```python
from build123d import *

# Parameters (mm, degrees)
SKETCH1_R           = 3.175
SKETCH1_R_2         = 1.325
BOSS_EXTRUDE1_DEPTH = 8


with BuildPart() as part:
    # Sketch1 → Boss-Extrude1 (new body)
    with BuildSketch(Plane.XY):
        with BuildLine():
            Line((-21.75, 27.5), (-6, 27.5))
            ThreePointArc((-6, 27.5), (0, 36.5), (6, 27.5))
            Line((6, 27.5), (21.75, 27.5))
            Line((21.75, 27.5), (21.75, 19.489664619))
            Line((21.75, 19.489664619), (37.852514493, 8.977148354))
            Line((37.852514493, 8.977148354), (59.375273358, 15.378390657))
            Line((59.375273358, 15.378390657), (64.476863532, 23.056267795))
            ThreePointArc((64.476863532, 23.056267795), (74.130822267, 30.891394037), (70.5, 19))
            Line((70.5, 19), (64.476863532, 8.759983115))
            Line((64.476863532, 8.759983115), (64.476863532, -8.759983115))
            Line((64.476863532, -8.759983115), (70.5, -19))
            ThreePointArc((70.5, -19), (74.130822267, -30.891394037), (64.476863532, -23.056267795))
            Line((64.476863532, -23.056267795), (59.375273358, -15.378390657))
            Line((59.375273358, -15.378390657), (37.852514493, -8.977148354))
            Line((37.852514493, -8.977148354), (21.75, -19.489664619))
            Line((21.75, -19.489664619), (21.75, -27.5))
            Line((21.75, -27.5), (6, -27.5))
            ThreePointArc((6, -27.5), (0, -36.5), (-6, -27.5))
            Line((-6, -27.5), (-21.75, -27.5))
            Line((-21.75, -27.5), (-21.75, -19.489664619))
            Line((-21.75, -19.489664619), (-37.852514493, -8.977148354))
            Line((-37.852514493, -8.977148354), (-59.375273358, -15.378390657))
            Line((-59.375273358, -15.378390657), (-64.476863532, -23.056267795))
            ThreePointArc((-64.476863532, -23.056267795), (-74.130822267, -30.891394037), (-70.5, -19))
            Line((-70.5, -19), (-64.476863532, -8.759983115))
            Line((-64.476863532, -8.759983115), (-64.476863532, 8.759983115))
            Line((-64.476863532, 8.759983115), (-70.5, 19))
            ThreePointArc((-70.5, 19), (-74.130822267, 30.891394037), (-64.476863532, 23.056267795))
            Line((-64.476863532, 23.056267795), (-59.375273358, 15.378390657))
            Line((-59.375273358, 15.378390657), (-37.852514493, 8.977148354))
            Line((-37.852514493, 8.977148354), (-21.75, 19.489664619))
            Line((-21.75, 19.489664619), (-21.75, 27.5))
        make_face()
        with Locations((0, 30)):
            Circle(SKETCH1_R, mode=Mode.SUBTRACT)
        with Locations((70.5, 25.5)):
            Circle(SKETCH1_R, mode=Mode.SUBTRACT)
        with Locations(Location((70.5, -25.5, 0), (0, 0, 180))):
            Circle(SKETCH1_R, mode=Mode.SUBTRACT)
        with Locations(Location((0, -30, 0), (0, 0, 180))):
            Circle(SKETCH1_R, mode=Mode.SUBTRACT)
        with Locations((-70.5, -25.5)):
            Circle(SKETCH1_R, mode=Mode.SUBTRACT)
        with Locations(Location((-70.5, 25.5, 0), (0, 0, 180))):
            Circle(SKETCH1_R, mode=Mode.SUBTRACT)
        with Locations((16.38, 21.46)):
            Circle(SKETCH1_R_2, mode=Mode.SUBTRACT)
        with Locations(Location((-16.38, 21.46, 0), (0, 0, 180))):
            Circle(SKETCH1_R_2, mode=Mode.SUBTRACT)
        with Locations((-16.38, -21.46)):
            Circle(SKETCH1_R_2, mode=Mode.SUBTRACT)
        with Locations(Location((16.38, -21.46, 0), (0, 0, 180))):
            Circle(SKETCH1_R_2, mode=Mode.SUBTRACT)
    extrude(amount=BOSS_EXTRUDE1_DEPTH)


solid = part.part
```
Work out the finished part from the listing and answer in its coordinate system (mm). A direction names the side the tool comes from. Give positions to 0.01 mm unless a question says otherwise; leave off trailing zeros. Loops run counter-clockwise (first coordinate to the right, second up) from the corner with the lowest first, then second, coordinate; pieces in that order, holes last. Notation, with made-up numbers: (71.5, -25) -> (99.5, -25) arc R20 ccw to (99.5, -11) -> close; hole circle Ø3 at (78, 18.25). An arc over 180 degrees is marked (long way). Write item = value, one per line. Start each with the question number.
(1) Find section B-B on z = 4. Give the number of separate pieces and of enclosed holes in the cut face, and give its area (3 significant figures).
(2) Find the intervals of material crossed by probe 1 along Y at (x, z) = (16.38, 6.75) (3 decimals); probe 2 along Y at (x, z) = (-70.5, 2) (3 decimals); probe 3 along X at (y, z) = (-29, 2.5), in increasing order. Write a range as from..to.
(3) Find section A-A on x = 0. Give the vertices of the cut face in (y, z) (3 decimals).
(4) The mould has two halves that part along Y. Classify faces 4 (the flat face through (-29.7, -14.3, 3.9)), 5 (the flat face through (1, 1, 8)), 6 (the flat face through (-67.53, -13.95, 3.94)), 7 (the flat face through (67.53, 13.95, 3.94)): +Y half, -Y half, draft (parallel to the pull), parting line (faces both ways), or undercut.
(5) Find section C-C on x = 35. Give the vertices of the cut face in (y, z), and give its area (3 significant figures).
(6) Given pin 1 Ø4 at (x, z) = (13, 2) entering from +Y; pin 2 Ø2 at (y, z) = (-19.5, 1) entering from +X; pin 3 Ø1.5 at (x, z) = (4, 5.5) entering from -Y, each flat-ended and moving along its own axis, determine where each tip first touches the part or whether it passes through.
(7) Which of the six approach directions +Z, -Z, +X, -X, +Y, -Y give full straight-line access (tool end or side, diameter ignored) to faces 1 (the flat face through (-48.46, -12.13, 3.94)), 2 (the flat face through (-48.76, 12.22, 3.94)), 3 (the cylindrical face through (-0.69, 26.9, 3.94))?
From the geometry:
q1.separate_pieces = 1
q1.enclosed_holes = 10
q1.area = 5,420 mm^2
q2.probe_1 = -27.5..-22.785, -20.135..20.135, 22.785..27.5
q2.probe_2 = -32..-28.675, -22.325..-19, 19..22.325, 28.675..32
q2.probe_3 = -75.98..-65.02, -6.42..-3.01, 3.01..6.42, 65.02..75.98
q3.outline = (-36.5, 0) -> (-33.175, 0) -> (-33.175, 8) -> (-36.5, 8) -> close; (-26.825, 0) -> (26.825, 0) -> (26.825, 8) -> (-26.825, 8) -> close; (33.175, 0) -> (36.5, 0) -> (36.5, 8) -> (33.175, 8) -> close
q4.face_4 = -Y half
q4.face_5 = draft
q4.face_6 = undercut
q4.face_7 = undercut
q5.outline = (-10.84, 0) -> (10.84, 0) -> (10.84, 8) -> (-10.84, 8) -> close
q5.area = 173 mm^2
q6.pin_1 = 27.5
q6.pin_2 = 74.65
q6.pin_3 = -35.63
q7.face_1 = +Z, -Z, -Y
q7.face_2 = +Z, -Z, +Y
q7.face_3 = +Z, -Z
